from build123d import *

# Parameters (mm, degrees)
SKETCH_1_W          = 40
SKETCH_1_H          = 42
SKETCH_1_R          = 2
SKETCH_1_R_2        = 17
EXTRUDE_1_DEPTH     = 3
EXTRUDE_2_DEPTH     = 20
CUT_EXTRUDE_1_DEPTH = 25
CUT_EXTRUDE_2_DEPTH = 4


with BuildPart() as part:
    # 草图1 → 凸台-拉伸1 (new body)
    with BuildSketch(Plane.XY):
        with Locations((-26.203389279, 21.300914244)):
            Rectangle(SKETCH_1_W, SKETCH_1_H)
        with Locations((-41.203389279, 34.800914244)):
            Circle(SKETCH_1_R, mode=Mode.SUBTRACT)
        with Locations((-11.203389279, 34.800914244)):
            Circle(SKETCH_1_R, mode=Mode.SUBTRACT)
        with Locations((-41.203389279, 4.800914244)):
            Circle(SKETCH_1_R, mode=Mode.SUBTRACT)
        with Locations((-11.203389279, 4.800914244)):
            Circle(SKETCH_1_R, mode=Mode.SUBTRACT)
        with Locations((-26.203389279, 19.800914244)):
            Circle(SKETCH_1_R_2, mode=Mode.SUBTRACT)
    extrude(amount=EXTRUDE_1_DEPTH)

    # 草图2 → 凸台-拉伸2 (add)
    with BuildSketch(Plane(origin=(0, 0, 0), x_dir=(-1, 0, 0), z_dir=(0, 0, -1))):
        Polygon((6.203389279, 42.300914244), (46.203389279, 42.300914244), (46.203389279, 0.300914244), (44.203389279, 0.300914244), (44.203389279, 39.300914244), (8.203389279, 39.300914244), (8.203389279, 0.300914244), (6.203389279, 0.300914244), align=None)
    extrude(amount=EXTRUDE_2_DEPTH)

    # 草图3 → 切除-拉伸1 (cut)
    with BuildSketch(Plane.XY.offset(3)):
        Polygon((-45.203389279, 42.300914244), (-46.203389279, 42.300914244), (-46.203389279, 41.300914244), align=None)
        Polygon((-6.203389279, 42.300914244), (-7.203389279, 42.300914244), (-6.203389279, 41.300914244), align=None)
        Polygon((-45.203389279, 0.300914244), (-46.203389279, 1.300914244), (-46.203389279, 0.300914244), align=None)
        Polygon((-6.203389279, 0.300914244), (-6.203389279, 1.300914244), (-7.203389279, 0.300914244), align=None)
    extrude(amount=-CUT_EXTRUDE_1_DEPTH, mode=Mode.SUBTRACT)

    # 草图5 → 切除-拉伸2 (cut)
    with BuildSketch(Plane(origin=(0, 42.300914244, 0), x_dir=(1, 0, 0), z_dir=(0, 1, 0))):
        with BuildLine():
            Line((-35.703389279, 7), (-35.703389279, 3))
            ThreePointArc((-35.703389279, 3), (-33.703389279, 1), (-31.703389279, 3))
            Line((-31.703389279, 3), (-31.703389279, 7))
            ThreePointArc((-31.703389279, 7), (-33.703389279, 9), (-35.703389279, 7))
        make_face()
        with BuildLine():
            Line((-20.703389279, 7), (-20.703389279, 3))
            ThreePointArc((-20.703389279, 3), (-18.703389279, 1), (-16.703389279, 3))
            Line((-16.703389279, 3), (-16.703389279, 7))
            ThreePointArc((-16.703389279, 7), (-18.703389279, 9), (-20.703389279, 7))
        make_face()
    extrude(amount=-CUT_EXTRUDE_2_DEPTH, mode=Mode.SUBTRACT)


solid = part.part
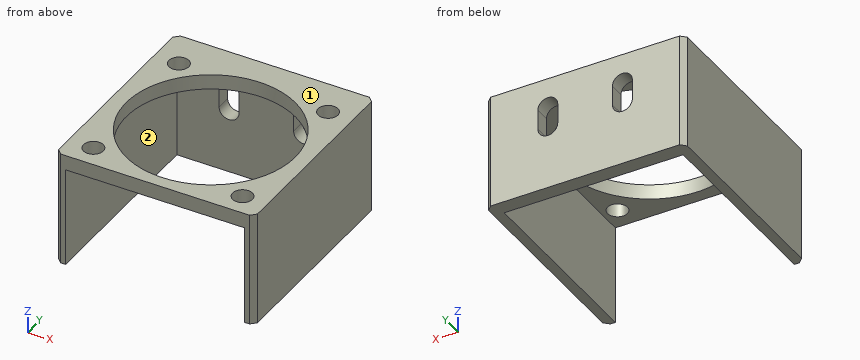
For this review, take the finished solid that the model builds, in its own axes (mm). Face numbers are marked on the shaded views. A direction names the side the tool comes from. Coordinates: 2 decimals unless noted, no trailing zeros. Write each loop counter-clockwise with the first axis right and the second up, starting at its lowest first coordinate (ties: lowest second). Pieces come first, ordered by that corner, then holes. Notation, with made-up numbers: (-21, 22) -> (19, 22) arc R8 ccw to (19, 37) -> close; hole circle Ø8 at (0.25, 49.5). An arc over 180 degrees is marked (long way). Write each question's results on one line, items separated by ' | '. Start each with the question number.
1) Consider section B-B (x = -12.5). Write out the cut boundary in (y, z), plus the area to 3 significant figures.
2) For the marked faces 1 and 2, list the 3-axis set-ups (+Z, -Z, +X, -X, +Y, -Y) from which the entire face can be reached by the end or side of a thin tool; tool diameter is ignored.
3) Consider section A-A (z = -5.75). Write out the cut boundary in (x, y).
4) Consider section C-C (z = 1.25). Write out the cut boundary in (x, y), plus the area to 3 significant figures.
5) Consider section D-D (x = -20). Write out the cut boundary in (y, z).
6) Insertion check: pin 1 (3 mm diameter, centred on x = -33.5, z = -14, fed in from -Y); pin 2 (4.5 mm diameter, centred on x = -11.2, y = 4.8, fed in from -Z). Each pin has a flat end and moves straight along its axis. Give the tip position at first contact, or say it passes through.
7) Wall thickness on L1, parallel to X at y = 23, z = -6.25; L2, parallel to Y at x = -10, z = -2.5; L3, parallel to Z at x = -11, y = 11.5: over which ranges is each line inside the solid? List them lowest first. Write a range as [from, to].
Geometry says:
1) outline: (0.3, 0) -> (3.28, 0) -> (3.28, 3) -> (0.3, 3) -> close; (6.32, 0) -> (9.74, 0) -> (9.74, 3) -> (6.32, 3) -> close; (29.86, 0) -> (33.28, 0) -> (33.28, 3) -> (29.86, 3) -> close; (36.32, 0) -> (39.3, 0) -> (39.3, -20) -> (42.3, -20) -> (42.3, 3) -> (36.32, 3) -> close | area: 107 mm^2
2) face 1: +Z, +X, -X, +Y, -Y | face 2: -Z, -Y
3) outline: (-46.2, 1.3) -> (-45.2, 0.3) -> (-44.2, 0.3) -> (-44.2, 39.3) -> (-35.7, 39.3) -> (-35.7, 42.3) -> (-45.2, 42.3) -> (-46.2, 41.3) -> close; (-31.7, 39.3) -> (-20.7, 39.3) -> (-20.7, 42.3) -> (-31.7, 42.3) -> close; (-16.7, 39.3) -> (-8.2, 39.3) -> (-8.2, 0.3) -> (-7.2, 0.3) -> (-6.2, 1.3) -> (-6.2, 41.3) -> (-7.2, 42.3) -> (-16.7, 42.3) -> close
4) outline: (-46.2, 1.3) -> (-45.2, 0.3) -> (-7.2, 0.3) -> (-6.2, 1.3) -> (-6.2, 41.3) -> (-7.2, 42.3) -> (-45.2, 42.3) -> (-46.2, 41.3) -> close; hole circle Ø4 at (-41.2, 4.8); hole circle Ø34 at (-26.2, 19.8); hole circle Ø4 at (-41.2, 34.8); hole circle Ø4 at (-11.2, 4.8); hole circle Ø4 at (-11.2, 34.8) | area: 720 mm^2
5) outline: (0.3, 0) -> (3.97, 0) -> (3.97, 3) -> (0.3, 3) -> close; (35.63, 0) -> (39.3, 0) -> (39.3, -1.48) -> (42.3, -1.48) -> (42.3, 3) -> (35.63, 3) -> close; (39.3, -20) -> (42.3, -20) -> (42.3, -8.52) -> (39.3, -8.52) -> close
6) pin 1: y = 39.3 | pin 2: z = 0
7) L1: [-46.2, -44.2], [-8.2, -6.2] | L2: [39.3, 42.3] | L3: [0, 3]
